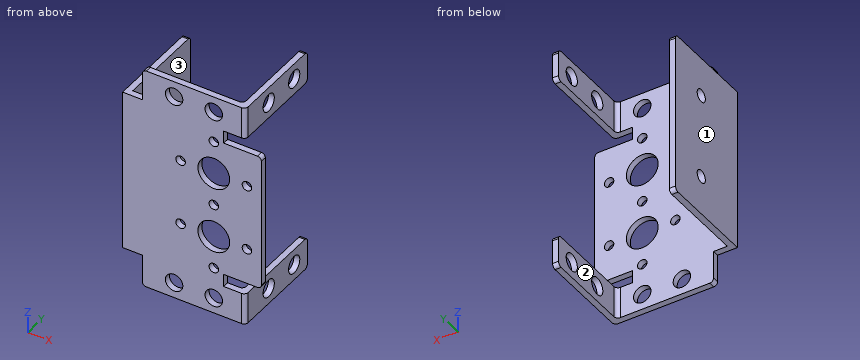
```python
from build123d import *

# Parameters (mm, degrees)
BOSS_EXTRUDE1_DEPTH = 57.2
SKETCH2_R           = 4
SKETCH2_R_2         = 2.2
SKETCH2_R_3         = 1.2
CUT_EXTRUDE1_DEPTH  = 72.325521379
SKETCH3_R           = 1.6
SKETCH3_W           = 8
SKETCH3_H           = 24.3
CUT_EXTRUDE3_DEPTH  = 5
CUT_EXTRUDE4_DEPTH  = 71.809233861
SKETCH5_W           = 1.5
SKETCH5_H           = 8
BOSS_EXTRUDE2_DEPTH = 22.74
FILLET1_R           = 1
SKETCH6_R           = 2.2
CUT_EXTRUDE5_DEPTH  = 5
FILLET2_R           = 1


with BuildPart() as part:
    # Sketch1 → Boss-Extrude1 (new body)
    with BuildSketch(Plane.XY):
        Polygon((0, 24.3), (1.56, 24.3), (1.56, 1.56), (35, 1.56), (35, 0), (0, 0), align=None)
    extrude(amount=-BOSS_EXTRUDE1_DEPTH)

    # Sketch2 → Cut-Extrude1 (cut, through all)
    with BuildSketch(Plane.XZ):
        with Locations(Location((23, -20.24, 0), (0, 0, 270))):
            Circle(SKETCH2_R)
        with Locations(Location((13, -53.25, 0), (0, 0, 180))):
            Circle(SKETCH2_R_2)
        with Locations(Location((23, -28.6, 0), (0, 0, 270))):
            Circle(SKETCH2_R_3)
        with Locations(Location((14.64, -20.24, 0), (0, 0, 270))):
            Circle(SKETCH2_R_3)
        with Locations(Location((23, -11.88, 0), (0, 0, 270))):
            Circle(SKETCH2_R_3)
        with Locations(Location((31.36, -20.24, 0), (0, 0, 270))):
            Circle(SKETCH2_R_3)
        with Locations(Location((23, -53.25, 0), (0, 0, 180))):
            Circle(SKETCH2_R_2)
        with Locations(Location((14.64, -36.96, 0), (0, 0, 180))):
            Circle(SKETCH2_R_3)
        with Locations(Location((31.36, -36.96, 0), (0, 0, 180))):
            Circle(SKETCH2_R_3)
        with Locations(Location((23, -3.95, 0), (0, 0, 270))):
            Circle(SKETCH2_R_2)
        with Locations(Location((23, -45.32, 0), (0, 0, 180))):
            Circle(SKETCH2_R_3)
        with Locations(Location((23, -36.96, 0), (0, 0, 180))):
            Circle(SKETCH2_R)
        with Locations(Location((13, -3.95, 0), (0, 0, 270))):
            Circle(SKETCH2_R_2)
    extrude(amount=-CUT_EXTRUDE1_DEPTH, mode=Mode.SUBTRACT)

    # Sketch3 → Cut-Extrude3 (cut)
    with BuildSketch(Plane.ZY):
        with Locations((-17.9, 14.2)):
            Circle(SKETCH3_R)
        with Locations(Location((-39.3, 14.2, 0), (0, 0, 90))):
            Circle(SKETCH3_R)
        with Locations((-4, 12.15)):
            Rectangle(SKETCH3_W, SKETCH3_H)
        with Locations((-53.2, 12.15)):
            Rectangle(SKETCH3_W, SKETCH3_H)
    extrude(amount=-CUT_EXTRUDE3_DEPTH, mode=Mode.SUBTRACT)

    # Sketch4 → Cut-Extrude4 (cut, through all)
    with BuildSketch(Plane(origin=(0, 1.56, 0), x_dir=(1, 0, 0), z_dir=(0, 1, 0))):
        Polygon((35, 57.2), (31, 57.2), (31, 49.2), (25.5, 49.2), (25.5, 46), (35, 46), align=None)
        Polygon((31, 8), (31, 0), (35, 0), (35, 11.2), (25.5, 11.2), (25.5, 8), align=None)
    extrude(amount=-CUT_EXTRUDE4_DEPTH, mode=Mode.SUBTRACT)

    # Sketch5 → Boss-Extrude2 (add)
    with BuildSketch(Plane(origin=(0, 1.56, 0), x_dir=(1, 0, 0), z_dir=(0, 1, 0))):
        with Locations((30.25, 53.2)):
            Rectangle(SKETCH5_W, SKETCH5_H)
        with Locations((30.25, 4)):
            Rectangle(SKETCH5_W, SKETCH5_H)
    extrude(amount=BOSS_EXTRUDE2_DEPTH)

    # Fillet1
    fillet1_edges = [part.edges().sort_by_distance(p)[0] for p in [
        (31, 0, -53.2),
        (31, 0, -4),
        (29.5, 1.56, -53.2),
        (29.5, 1.56, -4),
    ]]
    fillet(fillet1_edges, radius=FILLET1_R)

    # Sketch6 → Cut-Extrude5 (cut)
    with BuildSketch(Plane(origin=(31, 0, 0), x_dir=(0, 0, -1), z_dir=(1, 0, 0))):
        with Locations((4, 19.1)):
            Circle(SKETCH6_R)
        with Locations((4, 9.1)):
            Circle(SKETCH6_R)
        with Locations((53.2, 9.1)):
            Circle(SKETCH6_R)
        with Locations((53.2, 19.1)):
            Circle(SKETCH6_R)
    extrude(amount=-CUT_EXTRUDE5_DEPTH, mode=Mode.SUBTRACT)

    # Fillet2
    fillet2_edges = [part.edges().sort_by_distance(p)[0] for p in [
        (5, 0.78, -57.2),
        (0.78, 24.3, -49.2),
        (35, 0.78, -46),
        (35, 0.78, -11.2),
        (30.25, 24.3, -57.2),
        (30.25, 24.3, -49.2),
        (30.25, 24.3, -8),
        (30.25, 24.3, 0),
        (5, 0.78, 0),
        (0.78, 24.3, -8),
    ]]
    fillet(fillet2_edges, radius=FILLET2_R)


solid = part.part
```
Part model, mm, in its own coordinate system. Face numbers are marked on the shaded views. A direction names the side the tool comes from. Coordinates: 2 decimals unless noted, no trailing zeros. Write each loop counter-clockwise with the first axis right and the second up, starting at its lowest first coordinate (ties: lowest second). Pieces come first, ordered by that corner, then holes.
Item 1: Slice it at B-B (y = 6). Write the cut outline in (x, z), and give its area (3 significant figures).
Item 2: Slice it at D-D (y = 17.5). Write the cut outline in (x, z), and give its area (3 significant figures).
Item 3: Pin check, flat tips, straight feed: pin 1 (2.5 mm diameter, centred on x = 13, z = -3.95, fed in from -Y); pin 2 (0.5 mm diameter, centred on y = 1, z = -47, fed in from +X); pin 3 (16.5 mm diameter, centred on x = 17.5, z = -28, fed in from +Y); pin 4 (4 mm diameter, centred on x = 1.5, y = 12.5, fed in from -Z). Stop position of each tip, or through.
Item 4: Slice it at A-A (z = -28.6). Write the cut outline in (x, y), and give its area (3 significant figures).
Item 5: Slice it at C-C (x = 23). Count the separate pieces of the cut face and the enclosed holes in it, and give its area (3 significant figures).
Item 6: Which spindle directions (+Z, -Z, +X, -X, +Y, -Y) get a long thin tool onto all of the face, cutting with end or side? Do the marked faces 1, 2 and 3. Say none if no direction does.
Item 7: Probe line 1 (Y direction, x = 30, z = -4); line 2 (Z direction, x = 30, y = 5.5); line 3 (X direction, y = 0.75, z = -3.95). List the from-to ranges inside material, lowest first.
Results found:
1. outline: (0, -49.2) - (1.56, -49.2) - (1.56, -8) - (0, -8) - close; (29.5, -57.2) - (31, -57.2) - (31, -49.2) - (29.5, -49.2) - close; (29.5, -8) - (31, -8) - (31, 0) - (29.5, 0) - close
1. area: 88.3 mm2
2. outline: (0, -49.2) - (1.56, -49.2) - (1.56, -8) - (0, -8) - close; (29.5, -57.2) - (31, -57.2) - (31, -54.71) - (29.5, -54.71) - close; (29.5, -51.69) - (31, -51.69) - (31, -49.2) - (29.5, -49.2) - close; (29.5, -8) - (31, -8) - (31, -5.51) - (29.5, -5.51) - close; (29.5, -2.49) - (31, -2.49) - (31, 0) - (29.5, 0) - close
2. area: 79.2 mm2
3. pin 1: passes through
3. pin 2: stops at x = 25.5
3. pin 3: stops at y = 1.56
3. pin 4: stops at z = -49.2
4. outline: (0, 0) - (21.8, 0) - (21.8, 1.56) - (1.56, 1.56) - (1.56, 24.3) - (0, 24.3) - close; (24.2, 0) - (35, 0) - (35, 1.56) - (24.2, 1.56) - close
4. area: 86.3 mm2
5. separate pieces: 8
5. enclosed holes: 0
5. area: 39.3 mm2
6. face 1: +Z, -Z, -X, +Y, -Y
6. face 2: +Z, -Z, -X, +Y
6. face 3: +Z, -Z, +X, +Y
7. line 1: y = 0 to 6.9, 11.3 to 16.9, 21.3 to 24.3
7. line 2: z = -57.2 to -49.2, -8 to 0
7. line 3: x = 5 to 10.8, 15.2 to 20.8, 25.2 to 30.97
